```python
from build123d import *

# Parameters (mm, degrees)
SKETCH1_R           = 1
BOSS_EXTRUDE1_DEPTH = 1.5
SKETCH1_3_R         = 1
BOSS_EXTRUDE2_DEPTH = 6.5


with BuildPart() as part:
    # Sketch1 → Boss-Extrude1 (new, symmetric)
    with BuildSketch(Plane.XY):
        with BuildLine():
            Line((6.1, -1.5), (-6.1, -1.5))
            ThreePointArc((-6.1, -1.5), (-7.6, 0), (-6.1, 1.5))
            Line((-6.1, 1.5), (6.1, 1.5))
            ThreePointArc((6.1, 1.5), (7.6, 0), (6.1, -1.5))
        make_face()
        Circle(SKETCH1_R, mode=Mode.SUBTRACT)
    extrude(amount=BOSS_EXTRUDE1_DEPTH, both=True)

    # Sketch1_3 → Boss-Extrude2 (add, symmetric)
    with BuildSketch(Plane.XY):
        with Locations(Location((-6.1, 0, 0), (0, 0, 180))):
            Circle(SKETCH1_3_R)
        with Locations(Location((6.1, 0, 0), (0, 0, 180))):
            Circle(SKETCH1_3_R)
        with Locations(Location((0, 0, 0), (0, 0, 180))):
            Circle(SKETCH1_3_R)
    extrude(amount=BOSS_EXTRUDE2_DEPTH, both=True)


solid = part.part
```
Input: part model. Units: mm. Frame: model coordinates. A direction names the side the tool comes from. Round coordinates to 2 decimals unless told otherwise and drop trailing zeros. Loops run counter-clockwise (first coordinate to the right, second up) from the corner with the lowest first, then second, coordinate; pieces in that order, holes last. Notation, with made-up numbers: M 55,32 L 63,32 A15 cw 63,55 Z; hole C 59,-17.75 d6. An arc over 180 degrees is marked long. Answer in a Markdown table with one row per item. Add a question column.
1. Section A-A (y = 0). Output: boundary loops of the cut face in (x, z), and give its area (3 significant figures).
2. Mould query, pull axis X, two halves, no side actions, for faces 1 (the face through (-6, 0, 6.5)), 2 (the face through (0, 1, -4)), 3 (the face through (-7.6, 0, 0)). Classes: released by +X, released by -X, zero draft, split by the parting line, or undercut.
3. Section D-D (x = 5.75). Output: boundary loops of the cut face in (y, z).
4. Contact query for flat-ended pins moving along their axis: pin 1 (0.9 mm diameter, centred on x = 3, y = -0.5, fed in from -Z); pin 2 (0.9 mm diameter, centred on x = 1.5, y = 0.5, fed in from +Z). Output: stop coordinate, or through.
5. Ray query, probe 1 along X at (y, z) = (0.2, 5.75); probe 2 along X at (y, z) = (0.75, -5.5); probe 3 along Z at (x, y) = (1.75, 1.35). Return the intervals inside material, ascending.
6. Set-up query: faces 4 (the face through (0, 1, 4)), 5 (the face through (5.146, -0.3, -3.965)), 6 (the face through (0, 0, -6.5)). Return all of +Z, -Z, +X, -X, +Y, -Y with unobstructed straight access to the full face (end or side cutting, diameter ignored); none if empty.
7. Section C-C (z = 5). Output: boundary loops of the cut face in (x, y).
8. Section B-B (x = 0). Output: boundary loops of the cut face in (y, z), and give its area (3 significant figures).
Values follow:
| question | item | result |
|---|---|---|
| 1 | outline | M -7.6,-1.5 L -7.1,-1.5 L -7.1,-6.5 L -5.1,-6.5 L -5.1,-1.5 L -1,-1.5 L -1,-6.5 L 1,-6.5 L 1,-1.5 L 5.1,-1.5 L 5.1,-6.5 L 7.1,-6.5 L 7.1,-1.5 L 7.6,-1.5 L 7.6,1.5 L 7.1,1.5 L 7.1,6.5 L 5.1,6.5 L 5.1,1.5 L 1,1.5 L 1,6.5 L -1,6.5 L -1,1.5 L -5.1,1.5 L -5.1,6.5 L -7.1,6.5 L -7.1,1.5 L -7.6,1.5 Z |
| 1 | area | 106 mm^2 |
| 2 | face 1 | zero draft |
| 2 | face 2 | undercut |
| 2 | face 3 | released by -X |
| 3 | outline | M -1.5,-1.5 L -0.94,-1.5 L -0.94,-6.5 L 0.94,-6.5 L 0.94,-1.5 L 1.5,-1.5 L 1.5,1.5 L 0.94,1.5 L 0.94,6.5 L -0.94,6.5 L -0.94,1.5 L -1.5,1.5 Z |
| 4 | pin 1 | z = -1.5 |
| 4 | pin 2 | z = 1.5 |
| 5 | probe 1 | -7.08 to -5.12, -0.98 to 0.98, 5.12 to 7.08 |
| 5 | probe 2 | -6.76 to -5.44, -0.66 to 0.66, 5.44 to 6.76 |
| 5 | probe 3 | -1.5 to 1.5 |
| 6 | face 4 | +Z |
| 6 | face 5 | -Z |
| 6 | face 6 | -Z, +X, -X, +Y, -Y |
| 7 | outline | C -6.1,0 d2; C 0,0 d2; C 6.1,0 d2 |
| 8 | outline | M -1.5,-1.5 L -1,-1.5 L -1,-6.5 L 1,-6.5 L 1,-1.5 L 1.5,-1.5 L 1.5,1.5 L 1,1.5 L 1,6.5 L -1,6.5 L -1,1.5 L -1.5,1.5 Z |
| 8 | area | 29.0 mm^2 |
